Build history of the part. All positions in model axes, mm. Face numbers are marked on the shaded views. A direction names the side the tool comes from. Round coordinates to 2 decimals unless told otherwise and drop trailing zeros. Write each loop counter-clockwise with the first axis right and the second up, starting at its lowest first coordinate (ties: lowest second). Pieces come first, ordered by that corner, then holes. Notation, with made-up numbers: (69, 27.25) -> (123, 27.25) arc R20 cw to (123, 64.25) -> close; hole circle Ø1 at (-37.5, -23). An arc over 180 degrees is marked (long way). One line per question, with ' | ' between items.
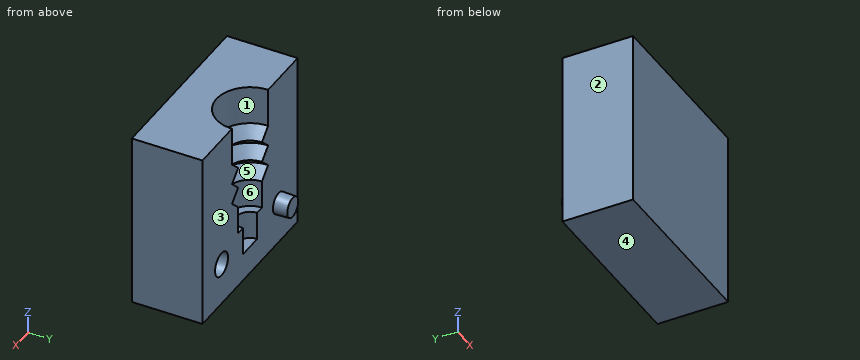
from build123d import *

# Parameters (mm, degrees)
SKETCH2_W           = 25
SKETCH2_H           = 25
BOSS_EXTRUDE1_DEPTH = 10
SKETCH4_R           = 1.5
BOSS_EXTRUDE2_DEPTH = 2
BOSS_EXTRUDE2_TAPER = 2
SKETCH5_R           = 1.7
CUT_EXTRUDE1_DEPTH  = 2.5


with BuildPart() as part:
    # Sketch2 → Boss-Extrude1 (new body)
    with BuildSketch(Plane(origin=(0, 0, 0), x_dir=(1, 0, 0), z_dir=(0, 1, 0))):
        Rectangle(SKETCH2_W, SKETCH2_H)
    extrude(amount=BOSS_EXTRUDE1_DEPTH)

    # Sketch3 → Cut-Revolve1 (revolve, cut)
    with BuildSketch(Plane(origin=(0, 10, 0), x_dir=(1, 0, 0), z_dir=(0, 1, 0))):
        Polygon((0, -12.5), (4.75, -12.5), (4.75, -7), (3.125, -5.5), (4.75, -4), (3.125, -2.5), (4.75, -1), (3.125, 0.5), (3.125, 4.5), (1.875, 4.5), (1.875, 8.5), (0, 8.5), align=None)
    revolve(axis=Axis((0, 10, -12.5), (0, 0, 1)), mode=Mode.SUBTRACT)

    # Sketch4 → Boss-Extrude2 (add)
    with BuildSketch(Plane(origin=(0, 10, 0), x_dir=(1, 0, 0), z_dir=(0, 1, 0))):
        with Locations((-7.5, 6.5)):
            Circle(SKETCH4_R)
    extrude(amount=BOSS_EXTRUDE2_DEPTH, taper=BOSS_EXTRUDE2_TAPER)

    # Sketch5 → Cut-Extrude1 (cut)
    with BuildSketch(Plane(origin=(0, 10, 0), x_dir=(1, 0, 0), z_dir=(0, 1, 0))):
        with Locations((7.5, 6.5)):
            Circle(SKETCH5_R)
    extrude(amount=-CUT_EXTRUDE1_DEPTH, mode=Mode.SUBTRACT)


solid = part.part
(1) Slice it at C-C (x = 7.5). Write the cut outline in (y, z), then the cut area to 4 significant figures.
Calculated:
outline: (0, -12.5) -> (10, -12.5) -> (10, -8.2) -> (7.5, -8.2) -> (7.5, -4.8) -> (10, -4.8) -> (10, 12.5) -> (0, 12.5) -> close | area: 241.5 mm2
(2) Slice it at B-B (z = -1.5). Write the cut outline in (x, y) (3 decimals), then the cut area to 3 significant figures.
Calculated:
outline: (-12.5, 0) -> (12.5, 0) -> (12.5, 10) -> (3.125, 10) arc R3.125 cw to (-3.125, 10) -> (-12.5, 10) -> close | area: 235 mm2
(3) 3-axis set-ups, long thin cutter, end or side, ignore diameter. For the marked faces 4, 5 and 6: which of +Z, -Z, +X, -X, +Y, -Y reach the whole face in a straight line?
Calculated:
face 4: -Z, +X, -X, +Y, -Y | face 5: +Y | face 6: +Z, +Y
(4) Wall check: line 1 (Z direction, x = 7.5, y = 8.65); line 2 (X direction, y = 9, z = -6.5); line 3 (X direction, y = 8.5, z = -6.5) (3 decimals). Give the ranges that are in metal, low to high. Write a range as from..to.
Calculated:
line 1: -12.5..-8.2, -4.8..12.5 | line 2: -12.5..-1.59, 1.59..5.8, 9.2..12.5 | line 3: -12.5..-1.125, 1.125..5.8, 9.2..12.5
(5) Drop flat-ended pins along their axis: pin 1 (0.9 mm diameter, centred on x = -0.5, y = 9, fed in from +Z); pin 2 (2.5 mm diameter, centred on x = 7, z = -6, fed in from +Y); pin 3 (0.9 mm diameter, centred on x = 0.5, y = 8, fed in from +Z). Give the stop position or say it passes through.
Calculated:
pin 1: z = -8.5 | pin 2: y = 10 | pin 3: z = -4.5
(6) Slice it at A-A (x = -7.5). Write the cut outline in (y, z), then the cut area to 3 significant figures.
Calculated:
outline: (0, -12.5) -> (10, -12.5) -> (10, -8) -> (12, -7.93) -> (12, -5.07) -> (10, -5) -> (10, 12.5) -> (0, 12.5) -> close | area: 256 mm2
(7) Mould opens along X. For the marked faces 1, 2 and 3 say: pulls with the +X half, pulls with the -X half, needs draft (parallel to the pull), parting line crosses it, or undercut.
Calculated:
face 1: undercut | face 2: pulls with the -X half | face 3: needs draft
(8) Slice it at D-D (z = 10.25). Write the cut outline in (x, y), then the cut area to 3 significant figures.
Calculated:
outline: (-12.5, 0) -> (12.5, 0) -> (12.5, 10) -> (4.75, 10) arc R4.75 cw to (-4.75, 10) -> (-12.5, 10) -> close | area: 215 mm2
